Source: CAD feature listing. Evaluate the final solid. Frame: model axes, mm. Round coordinates to 2 decimals unless told otherwise and drop trailing zeros. Answer as CSV lines item,"result". Start each with the question number.
Item 1: Line query: line 1 (Y direction, x = 165.5, z = 2.75); line 2 (Y direction, x = 169, z = 14.5); line 3 (X direction, y = 631.5, z = 11). Output: solid intervals per line, ascending. Write a range as [from, to].
Item 2: First-contact query: P1, Ø5, axis at x = 486.5, y = 737, coming from the -Z side (3 decimals). Flat tip, straight axial feed; report the tip coordinate or a pass-through.
Item 3: Section query A-A on z = 11.5. State how many separate pieces and enclosed holes the cut face has, plus the area to 3 significant figures.
from build123d import *

# Parameters (mm, degrees)
F0_W     = 1104.9
F0_H     = 2438.4
F1_DEPTH = 19.05
F3_DEPTH = 3.175
F5_DEPTH = 25.4


with BuildPart() as f1:
    # F0 (on Top) → F1 (new body)
    with BuildSketch(Plane.XY):
        with Locations((609.6, 1219.2)):
            Rectangle(F0_W, F0_H)
    extrude(amount=F1_DEPTH)

    # F2 (on Top) → F3 (cut)
    with BuildSketch(Plane.XY):
        with BuildLine():
            Line((180.975, 52.3875), (180.975, 369.8875))
            ThreePointArc((180.975, 369.8875), (166.6875, 384.175), (152.4, 369.8875))
            Line((152.4, 369.8875), (152.4, 52.3875))
            ThreePointArc((152.4, 52.3875), (166.6875, 38.1), (180.975, 52.3875))
        make_face()
        with BuildLine():
            ThreePointArc((1066.8, 369.8875), (1052.5125, 384.175), (1038.225, 369.8875))
            Line((1038.225, 369.8875), (1038.225, 52.3875))
            ThreePointArc((1038.225, 52.3875), (1052.5125, 38.1), (1066.8, 52.3875))
            Line((1066.8, 52.3875), (1066.8, 369.8875))
        make_face()
        with BuildLine():
            Line((482.6, 369.8875), (482.6, 52.3875))
            ThreePointArc((482.6, 52.3875), (496.8875, 38.1), (511.175, 52.3875))
            Line((511.175, 52.3875), (511.175, 369.8875))
            ThreePointArc((511.175, 369.8875), (496.8875, 384.175), (482.6, 369.8875))
        make_face()
        with BuildLine():
            ThreePointArc((736.6, 369.8875), (722.3125, 384.175), (708.025, 369.8875))
            Line((708.025, 369.8875), (708.025, 52.3875))
            ThreePointArc((708.025, 52.3875), (722.3125, 38.1), (736.6, 52.3875))
            Line((736.6, 52.3875), (736.6, 369.8875))
        make_face()
        with BuildLine():
            ThreePointArc((152.4, 550.8625), (166.6875, 536.575), (180.975, 550.8625))
            Line((180.975, 550.8625), (180.975, 868.3625))
            ThreePointArc((180.975, 868.3625), (166.6875, 882.65), (152.4, 868.3625))
            Line((152.4, 868.3625), (152.4, 550.8625))
        make_face()
        with BuildLine():
            Line((152.4, 1366.8375), (152.4, 1049.3375))
            ThreePointArc((152.4, 1049.3375), (166.6875, 1035.05), (180.975, 1049.3375))
            Line((180.975, 1049.3375), (180.975, 1366.8375))
            ThreePointArc((180.975, 1366.8375), (166.6875, 1381.125), (152.4, 1366.8375))
        make_face()
        with BuildLine():
            ThreePointArc((152.4, 1547.8125), (166.6875, 1533.525), (180.975, 1547.8125))
            Line((180.975, 1547.8125), (180.975, 1865.3125))
            ThreePointArc((180.975, 1865.3125), (166.6875, 1879.6), (152.4, 1865.3125))
            Line((152.4, 1865.3125), (152.4, 1547.8125))
        make_face()
        with BuildLine():
            ThreePointArc((511.175, 1865.3125), (496.8875, 1879.6), (482.6, 1865.3125))
            Line((482.6, 1865.3125), (482.6, 1547.8125))
            ThreePointArc((482.6, 1547.8125), (496.8875, 1533.525), (511.175, 1547.8125))
            Line((511.175, 1547.8125), (511.175, 1865.3125))
        make_face()
        with BuildLine():
            Line((1038.225, 868.3625), (1038.225, 550.8625))
            ThreePointArc((1038.225, 550.8625), (1052.5125, 536.575), (1066.8, 550.8625))
            Line((1066.8, 550.8625), (1066.8, 868.3625))
            ThreePointArc((1066.8, 868.3625), (1052.5125, 882.65), (1038.225, 868.3625))
        make_face()
        with BuildLine():
            Line((708.025, 868.3625), (708.025, 550.8625))
            ThreePointArc((708.025, 550.8625), (722.3125, 536.575), (736.6, 550.8625))
            Line((736.6, 550.8625), (736.6, 868.3625))
            ThreePointArc((736.6, 868.3625), (722.3125, 882.65), (708.025, 868.3625))
        make_face()
        with BuildLine():
            ThreePointArc((482.6, 550.8625), (496.8875, 536.575), (511.175, 550.8625))
            Line((511.175, 550.8625), (511.175, 868.3625))
            ThreePointArc((511.175, 868.3625), (496.8875, 882.65), (482.6, 868.3625))
            Line((482.6, 868.3625), (482.6, 550.8625))
        make_face()
        with BuildLine():
            ThreePointArc((708.025, 1049.3375), (722.3125, 1035.05), (736.6, 1049.3375))
            Line((736.6, 1049.3375), (736.6, 1366.8375))
            ThreePointArc((736.6, 1366.8375), (722.3125, 1381.125), (708.025, 1366.8375))
            Line((708.025, 1366.8375), (708.025, 1049.3375))
        make_face()
        with BuildLine():
            Line((708.025, 1865.3125), (708.025, 1547.8125))
            ThreePointArc((708.025, 1547.8125), (722.3125, 1533.525), (736.6, 1547.8125))
            Line((736.6, 1547.8125), (736.6, 1865.3125))
            ThreePointArc((736.6, 1865.3125), (722.3125, 1879.6), (708.025, 1865.3125))
        make_face()
        with BuildLine():
            Line((1038.225, 1865.3125), (1038.225, 1547.8125))
            ThreePointArc((1038.225, 1547.8125), (1052.5125, 1533.525), (1066.8, 1547.8125))
            Line((1066.8, 1547.8125), (1066.8, 1865.3125))
            ThreePointArc((1066.8, 1865.3125), (1052.5125, 1879.6), (1038.225, 1865.3125))
        make_face()
        with BuildLine():
            ThreePointArc((1038.225, 1049.3375), (1052.5125, 1035.05), (1066.8, 1049.3375))
            Line((1066.8, 1049.3375), (1066.8, 1366.8375))
            ThreePointArc((1066.8, 1366.8375), (1052.5125, 1381.125), (1038.225, 1366.8375))
            Line((1038.225, 1366.8375), (1038.225, 1049.3375))
        make_face()
        with BuildLine():
            Line((511.175, 1049.3375), (511.175, 1366.8375))
            ThreePointArc((511.175, 1366.8375), (496.8875, 1381.125), (482.6, 1366.8375))
            Line((482.6, 1366.8375), (482.6, 1049.3375))
            ThreePointArc((482.6, 1049.3375), (496.8875, 1035.05), (511.175, 1049.3375))
        make_face()
    extrude(amount=F3_DEPTH, mode=Mode.SUBTRACT)

    # F4 (on Top) → F5 (cut)
    with BuildSketch(Plane.XY):
        with BuildLine():
            Line((1048.0675, 356.309038), (1048.0675, 65.965962))
            ThreePointArc((1048.0675, 65.965962), (1052.5125, 38.1), (1056.9575, 65.965962))
            Line((1056.9575, 65.965962), (1056.9575, 356.309038))
            ThreePointArc((1056.9575, 356.309038), (1052.5125, 384.175), (1048.0675, 356.309038))
        make_face()
        with BuildLine():
            Line((726.7575, 65.965962), (726.7575, 356.309038))
            ThreePointArc((726.7575, 356.309038), (722.3125, 384.175), (717.8675, 356.309038))
            Line((717.8675, 356.309038), (717.8675, 65.965962))
            ThreePointArc((717.8675, 65.965962), (722.3125, 38.1), (726.7575, 65.965962))
        make_face()
        with BuildLine():
            Line((501.3325, 65.965962), (501.3325, 356.309038))
            ThreePointArc((501.3325, 356.309038), (496.8875, 384.175), (492.4425, 356.309038))
            Line((492.4425, 356.309038), (492.4425, 65.965962))
            ThreePointArc((492.4425, 65.965962), (496.8875, 38.1), (501.3325, 65.965962))
        make_face()
        with BuildLine():
            Line((171.1325, 65.965962), (171.1325, 356.309038))
            ThreePointArc((171.1325, 356.309038), (166.6875, 384.175), (162.2425, 356.309038))
            Line((162.2425, 356.309038), (162.2425, 65.965962))
            ThreePointArc((162.2425, 65.965962), (166.6875, 38.1), (171.1325, 65.965962))
        make_face()
        with BuildLine():
            Line((501.3325, 564.440962), (501.3325, 854.784038))
            ThreePointArc((501.3325, 854.784038), (496.8875, 882.65), (492.4425, 854.784038))
            Line((492.4425, 854.784038), (492.4425, 564.440962))
            ThreePointArc((492.4425, 564.440962), (496.8875, 536.575), (501.3325, 564.440962))
        make_face()
        with BuildLine():
            Line((717.8675, 854.784038), (717.8675, 564.440962))
            ThreePointArc((717.8675, 564.440962), (722.3125, 536.575), (726.7575, 564.440962))
            Line((726.7575, 564.440962), (726.7575, 854.784038))
            ThreePointArc((726.7575, 854.784038), (722.3125, 882.65), (717.8675, 854.784038))
        make_face()
        with BuildLine():
            Line((171.1325, 564.440962), (171.1325, 854.784038))
            ThreePointArc((171.1325, 854.784038), (166.6875, 882.65), (162.2425, 854.784038))
            Line((162.2425, 854.784038), (162.2425, 564.440962))
            ThreePointArc((162.2425, 564.440962), (166.6875, 536.575), (171.1325, 564.440962))
        make_face()
        with BuildLine():
            Line((1048.0675, 854.784038), (1048.0675, 564.440962))
            ThreePointArc((1048.0675, 564.440962), (1052.5125, 536.575), (1056.9575, 564.440962))
            Line((1056.9575, 564.440962), (1056.9575, 854.784038))
            ThreePointArc((1056.9575, 854.784038), (1052.5125, 882.65), (1048.0675, 854.784038))
        make_face()
        with BuildLine():
            Line((501.3325, 1062.915962), (501.3325, 1353.259038))
            ThreePointArc((501.3325, 1353.259038), (496.8875, 1381.125), (492.4425, 1353.259038))
            Line((492.4425, 1353.259038), (492.4425, 1062.915962))
            ThreePointArc((492.4425, 1062.915962), (496.8875, 1035.05), (501.3325, 1062.915962))
        make_face()
        with BuildLine():
            Line((717.8675, 1353.259038), (717.8675, 1062.915962))
            ThreePointArc((717.8675, 1062.915962), (722.3125, 1035.05), (726.7575, 1062.915962))
            Line((726.7575, 1062.915962), (726.7575, 1353.259038))
            ThreePointArc((726.7575, 1353.259038), (722.3125, 1381.125), (717.8675, 1353.259038))
        make_face()
        with BuildLine():
            Line((171.1325, 1062.915962), (171.1325, 1353.259038))
            ThreePointArc((171.1325, 1353.259038), (166.6875, 1381.125), (162.2425, 1353.259038))
            Line((162.2425, 1353.259038), (162.2425, 1062.915962))
            ThreePointArc((162.2425, 1062.915962), (166.6875, 1035.05), (171.1325, 1062.915962))
        make_face()
        with BuildLine():
            Line((1048.0675, 1353.259038), (1048.0675, 1062.915962))
            ThreePointArc((1048.0675, 1062.915962), (1052.5125, 1035.05), (1056.9575, 1062.915962))
            Line((1056.9575, 1062.915962), (1056.9575, 1353.259038))
            ThreePointArc((1056.9575, 1353.259038), (1052.5125, 1381.125), (1048.0675, 1353.259038))
        make_face()
        with BuildLine():
            Line((501.3325, 1561.390962), (501.3325, 1851.734038))
            ThreePointArc((501.3325, 1851.734038), (496.8875, 1879.6), (492.4425, 1851.734038))
            Line((492.4425, 1851.734038), (492.4425, 1561.390962))
            ThreePointArc((492.4425, 1561.390962), (496.8875, 1533.525), (501.3325, 1561.390962))
        make_face()
        with BuildLine():
            Line((717.8675, 1851.734038), (717.8675, 1561.390962))
            ThreePointArc((717.8675, 1561.390962), (722.3125, 1533.525), (726.7575, 1561.390962))
            Line((726.7575, 1561.390962), (726.7575, 1851.734038))
            ThreePointArc((726.7575, 1851.734038), (722.3125, 1879.6), (717.8675, 1851.734038))
        make_face()
        with BuildLine():
            Line((171.1325, 1561.390962), (171.1325, 1851.734038))
            ThreePointArc((171.1325, 1851.734038), (166.6875, 1879.6), (162.2425, 1851.734038))
            Line((162.2425, 1851.734038), (162.2425, 1561.390962))
            ThreePointArc((162.2425, 1561.390962), (166.6875, 1533.525), (171.1325, 1561.390962))
        make_face()
        with BuildLine():
            Line((1048.0675, 1851.734038), (1048.0675, 1561.390962))
            ThreePointArc((1048.0675, 1561.390962), (1052.5125, 1533.525), (1056.9575, 1561.390962))
            Line((1056.9575, 1561.390962), (1056.9575, 1851.734038))
            ThreePointArc((1056.9575, 1851.734038), (1052.5125, 1879.6), (1048.0675, 1851.734038))
        make_face()
    extrude(amount=F5_DEPTH, mode=Mode.SUBTRACT)


solid = f1.part
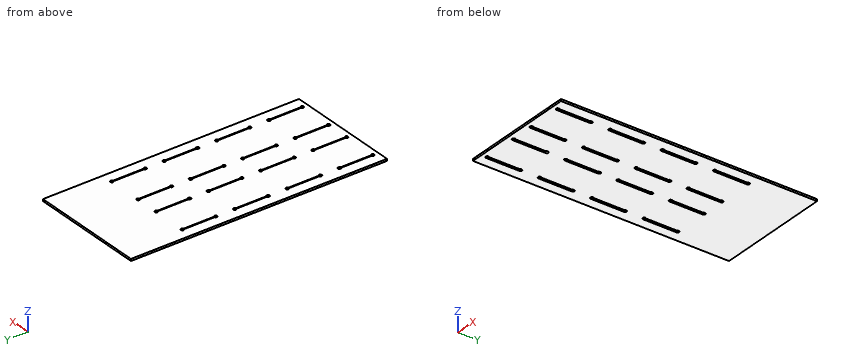
Results:
1,line 1,"[0, 38.15], [384.13, 536.62], [882.6, 1035.1], [1381.08, 1533.57], [1879.55, 2438.4]"
1,line 2,"[0, 38.29], [383.99, 536.76], [882.46, 1035.24], [1380.94, 1533.71], [1879.41, 2438.4]"
1,line 3,"[57.15, 162.24], [171.13, 492.44], [501.33, 717.87], [726.76, 1048.07], [1056.96, 1162.05]"
2,P1,"z = 3.175"
3,separate pieces,"1"
3,enclosed holes,"16"
3,area,"2,630,000 mm^2"
